Input: part model. Units: mm. Frame: model coordinates. Face numbers are marked on the shaded views. Coordinates: 2 decimals unless noted, no trailing zeros. Order: outer loops, then holes, each group sorted by start corner. A loop starts at its lowest first (then second) coordinate and runs counter-clockwise, first axis right, second up.
from build123d import *

# Parameters (mm, degrees)
F0_W     = 30
F0_H     = 10
F0_H_2   = 4
F0_H_3   = 2
F1_DEPTH = 2
F2_DEPTH = 5
F0_H_4   = 64
F3_DEPTH = 2


with BuildPart() as f1:
    # F0 (on Top) → F1 (new body)
    with BuildSketch(Plane.XY):
        with Locations((0, 47)):
            Rectangle(F0_W, F0_H)
        Polygon((15, -42), (15, -52), (25, -52), (25, 52), (15, 52), (15, 42), (15, 32), (15, -32), align=None)
        with Locations((0, 54)):
            Rectangle(F0_W, F0_H_2)
        with Locations((0, 57)):
            Rectangle(F0_W, F0_H_3)
        Polygon((-25, -52), (-15, -52), (-15, -42), (-15, -32), (-15, 32), (-15, 42), (-15, 52), (-25, 52), align=None)
    extrude(amount=F1_DEPTH)

    # F0 (on Top) → F2, piece 2 (join)
    with BuildSketch(Plane.XY):
        with Locations((0, 57)):
            Rectangle(F0_W, F0_H_3)
    extrude(amount=F2_DEPTH)



with BuildPart() as f1b:
    # F0 (on Top) → F1, piece 2 (new body)
    with BuildSketch(Plane.XY):
        with Locations((0, -54)):
            Rectangle(F0_W, F0_H_2)
        with Locations((0, -57)):
            Rectangle(F0_W, F0_H_3)
    extrude(amount=F1_DEPTH)

    # F0 (on Top) → F2 (join)
    with BuildSketch(Plane.XY):
        with Locations((0, -57)):
            Rectangle(F0_W, F0_H_3)
    extrude(amount=F2_DEPTH)


with BuildPart() as f1_1:
    add(f1.part)

    add(f1b.part)  # F3 merges F1b
    # F0 (on Top) → F3 (join)
    with BuildSketch(Plane.XY):
        Rectangle(F0_W, F0_H_4)
        with Locations((0, -47)):
            Rectangle(F0_W, F0_H)
    extrude(amount=F3_DEPTH)


solid = f1_1.part
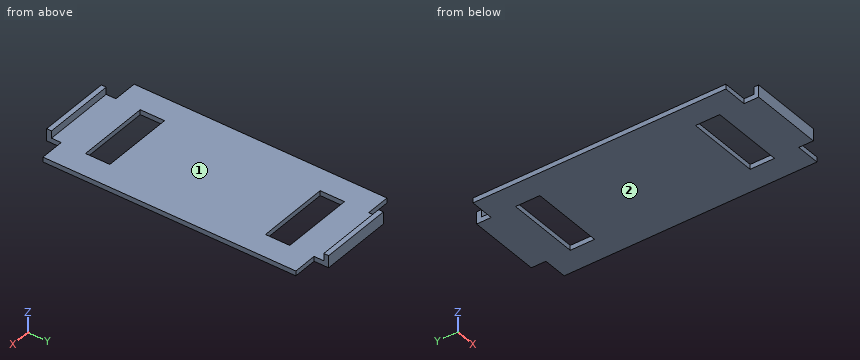
Item 1: Draft query along Y for the marked faces 1 and 2. Return one class per face: pulls with the +Y half, pulls with the -Y half, needs draft (parallel to the pull), parting line crosses it, or undercut.
Response values:
face 1: undercut
face 2: needs draft
Item 2: Ray query, probe 1 along Y at (x, z) = (-2, 1.55); probe 2 along Y at (x, z) = (7, 2.6); probe 3 along Y at (x, z) = (-17, 0.3). Return the intervals inside material, ascending.
Response values:
probe 1: y = -58 to -42, -32 to 32, 42 to 58
probe 2: y = -58 to -56, 56 to 58
probe 3: y = -52 to 52
Item 3: Cut plane B-B on y = -36. Return loops of the section in (x, z), then the cut area to 3 significant figures.
Response values:
outline: (-25, 0) - (-15, 0) - (-15, 2) - (-25, 2) - close; (15, 0) - (25, 0) - (25, 2) - (15, 2) - close
area: 40.0 mm2
Item 4: Cut plane C-C on x = 0.5. Return loops of the section in (y, z).
Response values:
outline: (-58, 0) - (-42, 0) - (-42, 2) - (-56, 2) - (-56, 5) - (-58, 5) - close; (-32, 0) - (32, 0) - (32, 2) - (-32, 2) - close; (42, 0) - (58, 0) - (58, 5) - (56, 5) - (56, 2) - (42, 2) - close
Item 5: Cut plane D-D on x = 17. Return loops of the section in (y, z).
Response values:
outline: (-52, 0) - (52, 0) - (52, 2) - (-52, 2) - close
Item 6: Cut plane A-A on z = 4.15. Return loops of the section in (x, y), then the cut area to 3 significant figures.
Response values:
outline: (-15, -58) - (15, -58) - (15, -56) - (-15, -56) - close; (-15, 56) - (15, 56) - (15, 58) - (-15, 58) - close
area: 120 mm2
Item 7: Pin query (flat end, axial travel): pin 1 Ø1.5 at (y, z) = (56, 3) entering from -X; pin 2 Ø5 at (x, y) = (10.5, -6.5) entering from +Z; pin 3 Ø2 at (x, z) = (20, 1) entering from -Y. Return the tip coordinate at first contact, or that it passes through.
Response values:
pin 1: stops at x = -15
pin 2: stops at z = 2
pin 3: stops at y = -52
